from build123d import *

# Parameters (mm, degrees)
F0_W     = 150
F0_H     = 55
F1_DEPTH = 22
F3_D     = 6.6
F4_D     = 28


with BuildPart() as f1:
    # F0 (on Top) → F1 (new body)
    with BuildSketch(Plane.XY):
        Rectangle(F0_W, F0_H)
    extrude(amount=F1_DEPTH)

    # F3 (through all)
    with Locations(Plane.XY.offset(22)):
        with Locations((-52.5, 20), (52.5, 20)):
            Hole(F3_D / 2)

    # F4 (through all)
    with Locations(Plane(origin=(0, 0, 0), x_dir=(1, 0, 0), z_dir=(0, 0, -1))):
        with Locations((0, 7.5)):
            Hole(F4_D / 2)


solid = f1.part
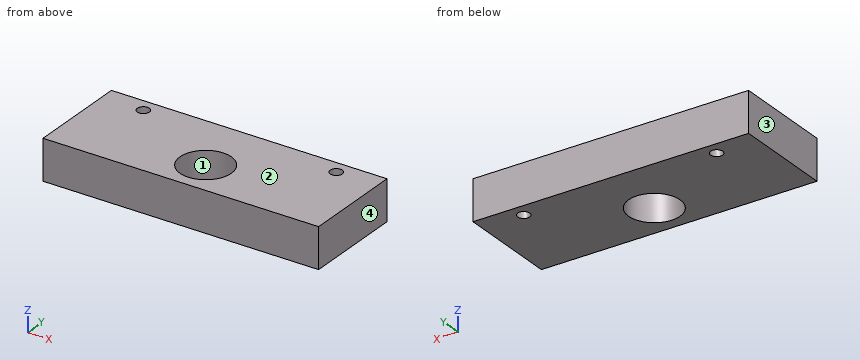
For this review, take the finished solid that the model builds, in its own axes (mm). Face numbers are marked on the shaded views. Round coordinates to 2 decimals unless told otherwise and drop trailing zeros. Write each loop counter-clockwise with the first axis right and the second up, starting at its lowest first coordinate (ties: lowest second). Pieces come first, ordered by that corner, then holes. Notation, with made-up numbers: M 50,59.25 L 104,59.25 A35 ccw 104,95.25 Z; hole C 89.25,35 d11. An arc over 180 degrees is marked long. Write item = value, one per line. Start each with the question number.
(1) We need section B-B (x = 0). Give the boundary of the cut face in (y, z), then the cut area to 3 significant figures.
(2) The part is to be moulded in two halves that separate along X. For the marked faces 1, 2, 3 and 4, say which applies: +X half, -X half, draft (parallel to the pull), parting line (faces both ways), or undercut.
(3) For line 1 along Y through (x, z) = (52.5, 8); line 2 along Y through (x, z) = (0, 12.25); line 3 along X through (y, z) = (-11, 13), list the stretches that pass through material, from the lowest coordinate up.
(4) We need section D-D (y = 20). Give the boundary of the cut face in (x, z).
(5) We need section A-A (y = -7.5). Give the boundary of the cut face in (x, z).
(6) We need section C-C (z = 19). Give the boundary of the cut face in (x, y), then the cut area to 3 significant figures.
Results found:
q1.outline = M -27.5,0 L -21.5,0 L -21.5,22 L -27.5,22 Z; M 6.5,0 L 27.5,0 L 27.5,22 L 6.5,22 Z
q1.area = 594 mm²
q2.face_1 = undercut
q2.face_2 = draft
q2.face_3 = -X half
q2.face_4 = +X half
q3.line_1 = -27.5 to 16.7, 23.3 to 27.5
q3.line_2 = -27.5 to -21.5, 6.5 to 27.5
q3.line_3 = -75 to -13.56, 13.56 to 75
q4.outline = M -75,0 L -55.8,0 L -55.8,22 L -75,22 Z; M -49.2,0 L 49.2,0 L 49.2,22 L -49.2,22 Z; M 55.8,0 L 75,0 L 75,22 L 55.8,22 Z
q5.outline = M -75,0 L -14,0 L -14,22 L -75,22 Z; M 14,0 L 75,0 L 75,22 L 14,22 Z
q6.outline = M -75,-27.5 L 75,-27.5 L 75,27.5 L -75,27.5 Z; hole C -52.5,20 d6.6; hole C 0,-7.5 d28; hole C 52.5,20 d6.6
q6.area = 7,570 mm²
